from build123d import *

# Parameters (mm, degrees)
SKETCH1_R           = 18.71
SKETCH1_R_2         = 1.1
SKETCH1_R_3         = 7.5
BOSS_EXTRUDE1_DEPTH = 2
SKETCH2_R           = 10
SKETCH2_R_2         = 7.5
BOSS_EXTRUDE2_DEPTH = 0.75


with BuildPart() as part:
    # Sketch1 → Boss-Extrude1 (new body)
    with BuildSketch(Plane.XY):
        Circle(SKETCH1_R)
        with Locations((0, -14.98)):
            Circle(SKETCH1_R_2, mode=Mode.SUBTRACT)
        with Locations((-12.973060549, 7.49)):
            Circle(SKETCH1_R_2, mode=Mode.SUBTRACT)
        with Locations((12.973060549, 7.49)):
            Circle(SKETCH1_R_2, mode=Mode.SUBTRACT)
        Circle(SKETCH1_R_3, mode=Mode.SUBTRACT)
    extrude(amount=BOSS_EXTRUDE1_DEPTH)

    # Sketch2 → Boss-Extrude2 (add)
    with BuildSketch(Plane.XY.offset(2)):
        Circle(SKETCH2_R)
        Circle(SKETCH2_R_2, mode=Mode.SUBTRACT)
    extrude(amount=BOSS_EXTRUDE2_DEPTH)


solid = part.part
Input: part model. Units: mm. Frame: model coordinates. A direction names the side the tool comes from. Give positions to 0.01 mm unless a question says otherwise; leave off trailing zeros. Order: outer loops, then holes, each group sorted by start corner. A loop starts at its lowest first (then second) coordinate and runs counter-clockwise, first axis right, second up. Notation, with made-up numbers: M 18.5,27 L 27.5,27 A31 cw 27.5,62 Z; hole C 85,-35 d8. An arc over 180 degrees is marked long. Answer as a JSON object with one key per item and string values.
1. Reachability of faces 1 (the flat face through (8, -8, 2)), 2 (the flat face through (4, 7, 2.75)) from +Z, -Z, +X, -X, +Y, -Y: full face, straight path, thin tool, end or side. Return the list, or none.
Result sheet:
{"face 1": "+Z", "face 2": "+Z, +X, -X, +Y, -Y"}
2. Cut plane A-A, the plane x = 0. Output: boundary loops of the cut face in (y, z).
Result sheet:
{"outline": "M -18.71,0 L -16.08,0 L -16.08,2 L -18.71,2 Z; M -13.88,0 L -7.5,0 L -7.5,2.75 L -10,2.75 L -10,2 L -13.88,2 Z; M 7.5,0 L 18.71,0 L 18.71,2 L 10,2 L 10,2.75 L 7.5,2.75 Z"}
3. Ray query, line 1 (Y direction, x = 0, z = 0.65); line 2 (Y direction, x = 0.5, z = 1.75); line 3 (Z direction, x = 7.5, y = -14). Return the intervals inside material, ascending. Write a range as [from, to].
Result sheet:
{"line 1": "[-18.71, -16.08], [-13.88, -7.5], [7.5, 18.71]", "line 2": "[-18.7, -15.96], [-14, -7.48], [7.48, 18.7]", "line 3": "[0, 2]"}
4. First-contact query: P1, Ø1, axis at y = -4.5, z = 2, coming from the +X side; P2, Ø10, axis at x = -15, y = -12, coming from the +Z side; P3, Ø1.5, axis at y = -4.5, z = 0.5, coming from the -X side. Flat tips, straight axial feed; report the tip coordinate or a pass-through.
Result sheet:
{"P1": "x = 18.28", "P2": "z = 2", "P3": "x = -18.33"}
5. Cut plane B-B, the plane y = 0. Output: boundary loops of the cut face in (x, z), and give its area (3 significant figures).
Result sheet:
{"outline": "M -18.71,0 L -7.5,0 L -7.5,2.75 L -10,2.75 L -10,2 L -18.71,2 Z; M 7.5,0 L 18.71,0 L 18.71,2 L 10,2 L 10,2.75 L 7.5,2.75 Z", "area": "48.6 mm²"}
6. Cut plane C-C, the plane z = 1.4. Output: boundary loops of the cut face in (x, y).
Result sheet:
{"outline": "C 0,0 d37.42; hole C -12.97,7.49 d2.2; hole C 0,0 d15; hole C 0,-14.98 d2.2; hole C 12.97,7.49 d2.2"}
7. Cut plane D-D, the plane x = -6.5. Output: boundary loops of the cut face in (y, z), and give its area (3 significant figures).
Result sheet:
{"outline": "M -17.54,0 L -3.74,0 L -3.74,2.75 L -7.6,2.75 L -7.6,2 L -17.54,2 Z; M 3.74,0 L 17.54,0 L 17.54,2 L 7.6,2 L 7.6,2.75 L 3.74,2.75 Z", "area": "61.0 mm²"}
8. Pull-direction query (Y, two-part tool) for faces 3 (the flat face through (0, -8, 0)), 4 (the cylindrical face through (12, 8, 1)), 5 (the cylindrical face through (-2.17, -9.76, 2.37)), 6 (the cylindrical face through (-7.493, 0.33, 1.356)); classes: +Y half, -Y half, draft (parallel to the pull), parting line (faces both ways), or undercut.
Result sheet:
{"face 3": "draft", "face 4": "undercut", "face 5": "parting line", "face 6": "undercut"}
